from build123d import *

# Parameters (mm, degrees)
F1_DEPTH = 12
F3_DEPTH = 25
F5_DEPTH = 25


with BuildPart() as f1:
    # F0 (on Front) → F1 (new body)
    with BuildSketch(Plane.XZ):
        Polygon((-1.5231755376, 71.0960855484), (-31.5231755376, 71.0960855484), (-31.5231755376, 9.5960855484), (-21.5231755376, 9.5960855484), (-21.5231755376, 66.0960855484), (-1.5231755376, 66.0960855484), align=None)
    extrude(amount=F1_DEPTH)

    # F2 (on face) → F3 (cut)
    with BuildSketch(Plane(origin=(-31.5231755376, 0, 0), x_dir=(0, -1, 0), z_dir=(-1, 0, 0))):
        with BuildLine():
            ThreePointArc((3.8, 16.0960855484), (6, 13.8960855484), (8.2, 16.0960855484))
            Line((8.2, 16.0960855484), (3.8, 16.0960855484))
        make_face()
        with BuildLine():
            Line((3.8, 16.0960855484), (8.2, 16.0960855484))
            ThreePointArc((8.2, 16.0960855484), (6, 18.2960855484), (3.8, 16.0960855484))
        make_face()
    extrude(amount=-F3_DEPTH, mode=Mode.SUBTRACT)

    # F4 (on face) → F5 (cut)
    with BuildSketch(Plane.XY.offset(71.0960855484)):
        with BuildLine():
            ThreePointArc((-9.3794432233, -4.7137606114), (-12.8094149262, -3.8562676857), (-13.6669078519, -7.2862393886))
            Line((-13.6669078519, -7.2862393886), (-9.3794432233, -4.7137606114))
        make_face()
        with BuildLine():
            Line((-9.3794432233, -4.7137606114), (-13.6669078519, -7.2862393886))
            ThreePointArc((-13.6669078519, -7.2862393886), (-10.8558415828, -8.4092873205), (-9.0231755376, -6))
            ThreePointArc((-9.0231755376, -6), (-9.1138882171, -5.3326660453), (-9.3794432233, -4.7137606114))
        make_face()
    extrude(amount=-F5_DEPTH, mode=Mode.SUBTRACT)


solid = f1.part
Can you work these out from the model? Positions are in its coordinate system, mm. A direction names the side the tool comes from. Give positions to 0.01 mm unless a question says otherwise; leave off trailing zeros. Loops run counter-clockwise (first coordinate to the right, second up) from the corner with the lowest first, then second, coordinate; pieces in that order, holes last. Notation, with made-up numbers: (12, -26.75) -> (47, -26.75) arc R15 cw to (47, -3.75) -> close; hole circle Ø11 at (-19, 24). An arc over 180 degrees is marked (long way). Write item = value, one per line.
1) For faces 4 (the flat face through (-21.523, -6, 37)), 5 (the flat face through (-27, -6, 9.596)), which set-ups out of +Z, -Z, +X, -X, +Y, -Y let a thin tool reach every point of the face, with its end or its side?
Check result:
face_4 = -Z, +X, +Y, -Y
face_5 = -Z, +X, -X, +Y, -Y
2) Suppose I cut it at A-A on x = -22.75. Write out the boundary of the cut face in (y, z).
Check result:
outline = (-12, 9.6) -> (0, 9.6) -> (0, 71.1) -> (-12, 71.1) -> close; hole circle Ø4.4 at (-6, 16.1)
3) Suppose I cut it at B-B on y = -1.75. Write out the boundary of the cut face in (x, z).
Check result:
outline = (-31.52, 9.6) -> (-21.52, 9.6) -> (-21.52, 66.1) -> (-1.52, 66.1) -> (-1.52, 71.1) -> (-31.52, 71.1) -> close
4) Thinking about a two-plate mould opening in Y: for faces 1 (the cylindrical face through (-26.593, -7.183, 17.951)), 2 (the flat face through (-16, -6, 71.096)), 3 (the flat face through (-23, -12, 48)), which applies, released by +Y, released by -Y, zero draft, split by the parting line, or undercut?
Check result:
face_1 = undercut
face_2 = zero draft
face_3 = released by -Y
5) I need wall thicknesses on L1, parallel to Z at x = -27.25, y = -6; L2, parallel to X at y = -1.5, z = 61; L3, parallel to Z at x = -19, y = -10.25. Which ranges of each line are inside material? Lowest first, please. Write a range as from..to.
Check result:
L1 = 9.6..13.9, 18.3..71.1
L2 = -31.52..-21.52
L3 = 66.1..71.1
6) Suppose I cut it at C-C on z = 37.5. Write out the boundary of the cut face in (x, y), then the cut area to 3 significant figures.
Check result:
outline = (-31.52, -12) -> (-21.52, -12) -> (-21.52, 0) -> (-31.52, 0) -> close
area = 120 mm2
7) Suppose I cut it at D-D on x = -7. Write out the boundary of the cut face in (y, z), then the cut area to 3 significant figures.
Check result:
outline = (-12, 66.1) -> (0, 66.1) -> (0, 71.1) -> (-12, 71.1) -> close
area = 60.0 mm2
8) Will these pins go through, and if not, where does the flat tip stop? pin 1 (6 mm diameter, centred on y = -7.5, z = 55, fed in from +X); pin 2 (3 mm diameter, centred on x = -19, z = 57, fed in from +Y); pin 3 (2 mm diameter, centred on x = -15.5, y = -2.5, fed in from -Z).
Check result:
pin_1 = -21.52
pin_2 = through
pin_3 = 66.1
